from build123d import *

# Parameters (mm, degrees)
SKETCH1_W                     = 185
SKETCH1_H                     = 80
BOSS_EXTRUDE1_DEPTH           = 12.7
M16_CLEARANCE_HOLE1_D         = 17
M6X1_0_START                  = -1
M6X1_0_TAPPED_HOLE2_OUTLINE_R = 2.5
M6X1_0_TAPPED_HOLE2_DEPTH     = 15
FILLET1_SIZE                  = 15
SKETCH5_R                     = 8
CUT_EXTRUDE1_DEPTH            = 102.575292414
M4_CLEARANCE_HOLE1_D          = 4.32


with BuildPart() as part:
    # Sketch1 → Boss-Extrude1 (new body)
    with BuildSketch(Plane(origin=(0, 0, 0), x_dir=(1, 0, 0), z_dir=(0, 1, 0))):
        Rectangle(SKETCH1_W, SKETCH1_H)
    extrude(amount=BOSS_EXTRUDE1_DEPTH)

    # M16 Clearance Hole1 (through all)
    with Locations(Plane(origin=(0, 12.7, 0), x_dir=(1, 0, 0), z_dir=(0, 1, 0))):
        with Locations((0, 0)):
            Hole(M16_CLEARANCE_HOLE1_D / 2)

    # M6x1.0 Tapped Hole2: read off the stored shape, not the designer's step
    # M6x1.0 Tapped Hole2 outline → M6x1.0 Tapped Hole2 (cut)
    with BuildSketch(Plane(origin=(0, 0, 0), x_dir=(1, 0, 0), z_dir=(0, 1, 0)).offset(M6X1_0_START)):
        with Locations((20, 20)):
            Circle(M6X1_0_TAPPED_HOLE2_OUTLINE_R)
        with Locations((-20, -20)):
            Circle(M6X1_0_TAPPED_HOLE2_OUTLINE_R)
        with Locations((20, -20)):
            Circle(M6X1_0_TAPPED_HOLE2_OUTLINE_R)
        with Locations((-20, 20)):
            Circle(M6X1_0_TAPPED_HOLE2_OUTLINE_R)
    extrude(amount=M6X1_0_TAPPED_HOLE2_DEPTH, mode=Mode.SUBTRACT)

    # Fillet1
    # a fillet whose section is not a circle: 15 mm, written as the material it takes off along each edge
    with BuildSketch(Plane(origin=(-92.5, -37.5, -40), x_dir=(1, 0, 0), z_dir=(0, 1, 0)), Plane(origin=(-92.5, -37.5, 40), x_dir=(0, 0, -1), z_dir=(0, 1, 0))) as fillet1_piece_1:
        with BuildLine():
            add(Edge.make_bspline([(FILLET1_SIZE, 0), (FILLET1_SIZE * 0.831801948466, 0), (FILLET1_SIZE * 0.663603896932, 0), (FILLET1_SIZE * 0.292893218813, -FILLET1_SIZE * 0.0716919198361), (FILLET1_SIZE * 0.0716919198361, -FILLET1_SIZE * 0.292893218813), (0, -FILLET1_SIZE * 0.663603896932), (0, -FILLET1_SIZE * 0.831801948466), (0, -FILLET1_SIZE)], knots=[0, 0, 0, 0, 0, 0, 0.5, 0.5, 1, 1, 1, 1, 1, 1], degree=5))
            Line((0, -FILLET1_SIZE), (0, 0))
            Line((0, 0), (FILLET1_SIZE, 0))
        make_face()
    extrude(amount=87.7, mode=Mode.SUBTRACT)
    with BuildSketch(Plane(origin=(92.5, -37.5, -40), x_dir=(-1, 0, 0), z_dir=(0, 1, 0)), Plane(origin=(92.5, -37.5, 40), x_dir=(0, 0, -1), z_dir=(0, 1, 0))) as fillet1_piece_2:
        with BuildLine():
            add(Edge.make_bspline([(FILLET1_SIZE, 0), (FILLET1_SIZE * 0.831801948466, 0), (FILLET1_SIZE * 0.663603896932, 0), (FILLET1_SIZE * 0.292893218813, FILLET1_SIZE * 0.0716919198361), (FILLET1_SIZE * 0.0716919198361, FILLET1_SIZE * 0.292893218813), (0, FILLET1_SIZE * 0.663603896932), (0, FILLET1_SIZE * 0.831801948466), (0, FILLET1_SIZE)], knots=[0, 0, 0, 0, 0, 0, 0.5, 0.5, 1, 1, 1, 1, 1, 1], degree=5))
            Line((0, FILLET1_SIZE), (0, 0))
            Line((0, 0), (FILLET1_SIZE, 0))
        make_face()
    extrude(amount=87.7, mode=Mode.SUBTRACT)

    # Sketch5 → Cut-Extrude1 (cut, through all)
    with BuildSketch(Plane(origin=(0, 12.7, 0), x_dir=(1, 0, 0), z_dir=(0, 1, 0))):
        with Locations(Location((-72, 0, 0), (0, 0, 270))):
            Circle(SKETCH5_R)
        with Locations(Location((72, 0, 0), (0, 0, 270))):
            Circle(SKETCH5_R)
    extrude(amount=-CUT_EXTRUDE1_DEPTH, mode=Mode.SUBTRACT)

    # M4 Clearance Hole1 (through all)
    with Locations(Plane(origin=(0, 0, 0), x_dir=(-1, 0, 0), z_dir=(0, -1, 0))):
        with Locations((60.686291501, 11.313708499), (72, 16), (83.313708499, 11.313708499), (60.686291501, -11.313708499), (72, -16), (83.313708499, -11.313708499), (-83.313708499, -11.313708499), (-72, -16), (-60.686291501, -11.313708499), (-60.686291501, 11.313708499), (-83.313708499, 11.313708499), (-72, 16)):
            Hole(M4_CLEARANCE_HOLE1_D / 2)


solid = part.part
Could you check a few things on this model? Use its own coordinates, in mm. Give positions to 0.01 mm unless a question says otherwise; leave off trailing zeros. Order: outer loops, then holes, each group sorted by start corner. A loop starts at its lowest first (then second) coordinate and runs counter-clockwise, first axis right, second up.
1. Suppose I cut it at A-A (x = -20). List the corners of the cut face in (y, z) for me.
2. Suppose I cut it at C-C (x = -72). List the corners of the cut face in (y, z) for me, plus the area to 3 significant figures.
3. Suppose I cut it at B-B (x = 4.5). List the corners of the cut face in (y, z) for me, plus the area to 3 significant figures.
4. Suppose I cut it at D-D (y = 9.5). Give the number of separate pieces and of enclosed holes in the cut face, plus the area to 3 significant figures.
5. I need wall thicknesses on L1, parallel to X at y = 10.25, z = 16; L2, parallel to X at y = 2, z = 11; L3, parallel to X at y = 7.75, z = -21. Which ranges of each line are inside material? Lowest first, please.
6. We'd pull the mould along X, two halves only. Please class faces 1 (the flat face through (-92.5, 6, 0)), 2 (the flat face through (-1, 0, -9)), 3 (the cylindrical face through (-84.91, 6.44, -12.77)): pulls with the +X half, pulls with the -X half, needs draft (parallel to the pull), parting line crosses it, or undercut.
Solved:
1. outline: (0, -40) - (12.7, -40) - (12.7, -22.5) - (0, -22.5) - close; (0, -17.5) - (12.7, -17.5) - (12.7, 17.5) - (0, 17.5) - close; (0, 22.5) - (12.7, 22.5) - (12.7, 40) - (0, 40) - close
2. outline: (0, -40) - (12.7, -40) - (12.7, -18.16) - (0, -18.16) - close; (0, -13.84) - (12.7, -13.84) - (12.7, -8) - (0, -8) - close; (0, 8) - (12.7, 8) - (12.7, 13.84) - (0, 13.84) - close; (0, 18.16) - (12.7, 18.16) - (12.7, 40) - (0, 40) - close
2. area: 703 mm2
3. outline: (0, -40) - (12.7, -40) - (12.7, -7.21) - (0, -7.21) - close; (0, 7.21) - (12.7, 7.21) - (12.7, 40) - (0, 40) - close
3. area: 833 mm2
4. separate pieces: 1
4. enclosed holes: 19
4. area: 13,800 mm2
5. L1: x = -92.5 to -74.16, -69.84 to 69.84, 74.16 to 92.5
5. L2: x = -92.5 to -85.45, -81.18 to -62.82, -58.55 to 58.55, 62.82 to 81.18, 85.45 to 92.5
5. L3: x = -92.5 to -22.29, -17.71 to 17.71, 22.29 to 92.5
6. face 1: pulls with the -X half
6. face 2: needs draft
6. face 3: undercut
